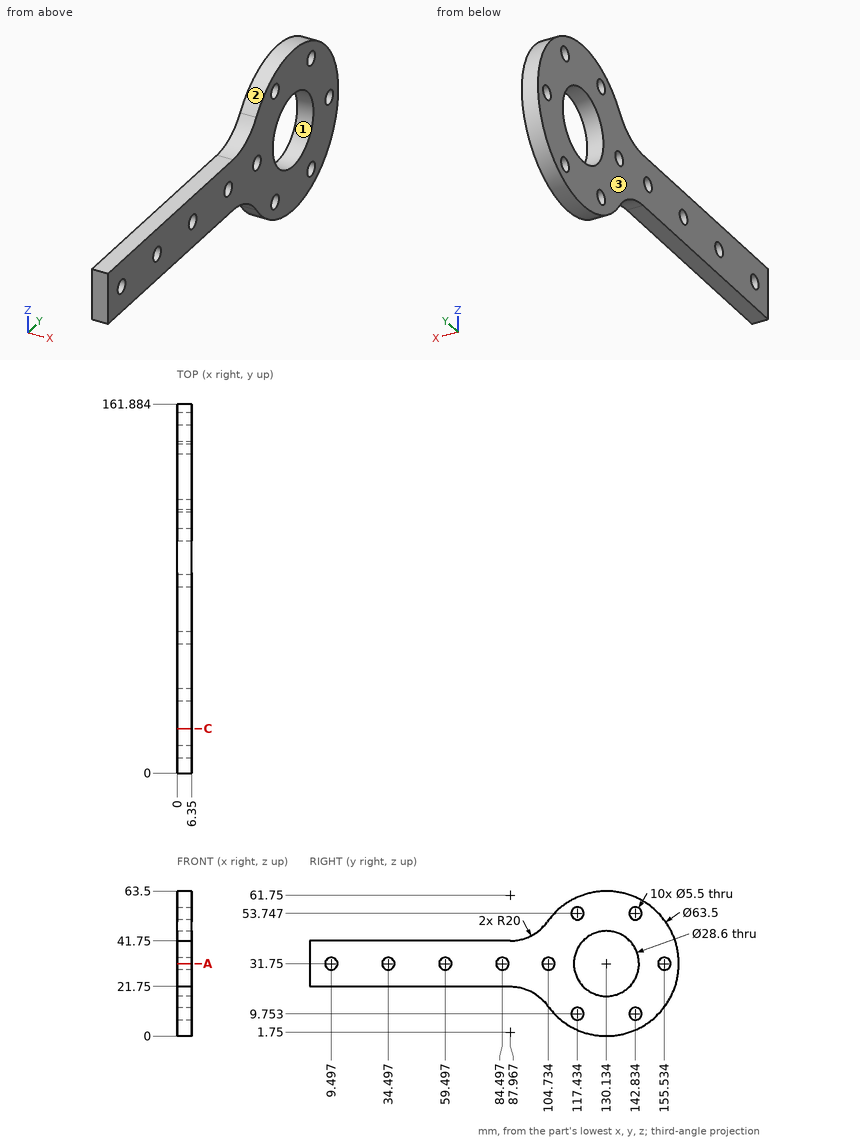
Design review of the part shown in the three views and the two pictorial views. Dimensions are in mm from the part's minimum x, y and z. Coordinates: 2 decimals unless noted, no trailing zeros. Loops run counter-clockwise (first coordinate to the right, second up) from the corner with the lowest first, then second, coordinate; pieces in that order, holes last.
Q1. We need section A-A on z = 31.75. State how many separate pieces and enclosed holes the cut face has, and give its area (3 significant figures).
Reported:
separate pieces: 8
enclosed holes: 0
area: 637 mm2
Q2. For pin 1 (3 mm diameter, centred on x = 5, z = 33.5, fed in from +Y); pin 2 (1.5 mm diameter, centred on x = 5.5, z = 7, fed in from +Y); pin 3 (3 mm diameter, centred on x = 3, y = 36.5, fed in from -Z), all flat-tipped, find the tip position at first contact; note any pin that passes through.
Reported:
pin 1: stops at y = 161.88
pin 2: stops at y = 150.92
pin 3: stops at z = 21.75
Q3. We need section C-C on y = 19.5. State the section outline as (x, z) points, and give its area (3 significant figures).
Reported:
outline: (0, 21.75) - (6.35, 21.75) - (6.35, 41.75) - (0, 41.75) - close
area: 127 mm2
Q4. The part is to be moulded in two halves that separate along Z. For the marked faces 1, 2 and 3, say which applies: +Z half, -Z half, draft (parallel to the pull), parting line (faces both ways), or undercut.
Reported:
face 1: undercut
face 2: parting line
face 3: draft
Q5. To check wall thickness, follow line 1 (Z direction, x = 0.5, y = 84.5); line 2 (Z direction, x = 2.5, y = 79); line 3 (Y direction, x = 1, z = 36). State the ranges of each line that lie inside material, in increasing order.
Reported:
line 1: z = 21.75 to 29, 34.5 to 41.75
line 2: z = 21.75 to 41.75
line 3: y = 0 to 116.48, 143.79 to 161.6
